Can you work these out from the model? Positions are in its coordinate system, mm. A direction names the side the tool comes from. Round coordinates to 2 decimals unless told otherwise and drop trailing zeros. Order: outer loops, then holes, each group sorted by start corner. A loop starts at its lowest first (then second) coordinate and runs counter-clockwise, first axis right, second up. Notation, with made-up numbers: M 3,26 L 26,26 A10 ccw 26,34 Z; hole C -27,-23 d5. An arc over 180 degrees is marked long. Answer as a JSON object with one key per item and string values. Group by question number.
```python
from build123d import *

# Parameters (mm, degrees)
BOSS_EXTRUDE1_DEPTH = 1.5
LPATTERN1_COUNT     = 2
LPATTERN1_PITCH     = 49
SKETCH2_W           = 50.5
SKETCH2_H           = 13
BOSS_EXTRUDE2_DEPTH = 1.5
SKETCH3_W           = 50.5
SKETCH3_H           = 6.5
BOSS_EXTRUDE3_DEPTH = 1.5


with BuildPart() as part:
    # Sketch1 → Boss-Extrude1 (new body)
    with BuildSketch(Plane(origin=(0, 0, 0), x_dir=(0, 0, -1), z_dir=(1, 0, 0))):
        with BuildLine():
            Line((0, 6.5), (0, -6.5))
            Line((0, -6.5), (-8.7, -6.5))
            ThreePointArc((-8.7, -6.5), (-11.245584412, -5.445584412), (-12.3, -2.9))
            Line((-12.3, -2.9), (-12.3, 2.9))
            ThreePointArc((-12.3, 2.9), (-11.245584412, 5.445584412), (-8.7, 6.5))
            Line((-8.7, 6.5), (0, 6.5))
        make_face()
    extrude(amount=BOSS_EXTRUDE1_DEPTH)


with BuildPart() as lpattern1_1:
    # LPattern1: pattern copy
    add(part.part.moved(Location(Vector(1, 0, 0) * (1 * LPATTERN1_PITCH))))


with BuildPart() as part_1:
    add(part.part)

    add(lpattern1_1.part)  # Boss-Extrude2 merges LPattern1_1
    # Sketch2 → Boss-Extrude2 (add)
    with BuildSketch(Plane.XY):
        with Locations((25.25, 0)):
            Rectangle(SKETCH2_W, SKETCH2_H)
    extrude(amount=BOSS_EXTRUDE2_DEPTH)

    # Sketch3 → Boss-Extrude3 (add)
    with BuildSketch(Plane.XZ.offset(6.5)):
        with Locations((25.25, 3.25)):
            Rectangle(SKETCH3_W, SKETCH3_H)
    boss_extrude3 = extrude(amount=-BOSS_EXTRUDE3_DEPTH)

    # Mirror1: Boss-Extrude3 across plane
    add(boss_extrude3.mirror(Plane.ZX))


solid = part_1.part
```
1) If we section it at D-D on z = 11: Write out the boundary of the cut face in (x, y).
2) Which directions (+Z, -Z, +X, -X, +Y, -Y) give clear straight access to the entire face, cutting with the end or side of a thin tool? Please do faces 1 (the face through (25, 6, 6.5)), 2 (the face through (25, 5, 4)), 3 (the face through (49.74, -5.47, 11.22)).
3) For pin 1 (1 mm diameter, centred on x = 36.5, y = -3.5, fed in from +Z); pin 2 (2 mm diameter, centred on x = 43.5, y = 4.5, fed in from +Z), each with a flat end and sliding along its axis, tell me the tip position at first contact or that it passes through.
4) If we section it at A-A on z = 4.25: Write out the boundary of the cut face in (x, y), plus the area to 4 significant figures.
5) If we section it at B-B on y = 0.5: Write out the boundary of the cut face in (x, z), plus the area to 3 significant figures.
6) If we section it at C-C on x = 37: Write out the boundary of the cut face in (y, z).
7) I need wall thicknesses on line 1 along Y through (x, z) = (25.5, 3.75); line 2 along X through (y, z) = (-1.5, 4.5); line 3 along Z through (x, y) = (24.5, -5.75). Which ranges of each line are inside material? Lowest first, please.
8) We'd pull the mould along Y, two halves only. Please class faces 4 (the face through (25, -6, 6.5)), 5 (the face through (25, -5, 4)), 6 (the face through (0.74, -5.47, 11.22)), 7 (the face through (1.5, 0, 7)): +Y half, -Y half, draft (parallel to the pull), parting line (faces both ways), or undercut.
Findings:
{
 "1": {"outline": "M 0,-5.67 L 1.5,-5.67 L 1.5,5.67 L 0,5.67 Z; M 49,-5.67 L 50.5,-5.67 L 50.5,5.67 L 49,5.67 Z"},
 "2": {"face 1": "+Z, +Y, -Y", "face 2": "+Z", "face 3": "+Z, +X, -X, -Y"},
 "3": {"pin 1": "stops at z = 1.5", "pin 2": "stops at z = 6.5"},
 "4": {"outline": "M 0,-6.5 L 50.5,-6.5 L 50.5,6.5 L 0,6.5 Z; hole M 1.5,-5 L 49,-5 L 49,5 L 1.5,5 Z", "area": "181.5 mm^2"},
 "5": {"outline": "M 0,0 L 50.5,0 L 50.5,12.3 L 49,12.3 L 49,1.5 L 1.5,1.5 L 1.5,12.3 L 0,12.3 Z", "area": "108 mm^2"},
 "6": {"outline": "M -6.5,0 L 6.5,0 L 6.5,6.5 L 5,6.5 L 5,1.5 L -5,1.5 L -5,6.5 L -6.5,6.5 Z"},
 "7": {"line 1": "y = -6.5 to -5, 5 to 6.5", "line 2": "x = 0 to 1.5, 49 to 50.5", "line 3": "z = 0 to 6.5"},
 "8": {"face 4": "draft", "face 5": "undercut", "face 6": "-Y half", "face 7": "undercut"}
}
